Autodesk Inventor part; units mm, degrees
ref_plane "YZ Plane" through (0, 0, 0) normal (1, 0, 0) x (0, 1, 0)
ref_plane "XZ Plane" through (0, 0, 0) normal (0, 1, 0) x (-1, 0, 0)
ref_plane "XY Plane" through (0, 0, 0) normal (0, 0, 1) x (1, 0, 0)
sketch "Sketch1" plane through (0, 0, 0) normal (0, 1, 0) x (-1, 0, 0)
  line L0 (-11, 8) -> (11, 8)
  line L1 (11, 8) -> (11, -8)
  line L2 (11, -8) -> (-11, -8)
  line L3 (-11, -8) -> (-11, 8)
  line L4 (-11, 8) -> (11, -8) construction
  line L5 (11, 8) -> (-11, -8) construction
  point P0 (0, 0)
  dimension "d0" = 22
  dimension "d1" = 16
extrude "Extrusion1" add sketch "Sketch1" along normal blind 13
sketch "Sketch2" plane through (11, 0, 8) normal (1, 0, 0) x (0, 0, -1)
  line L0 (1.5, 11.7761) -> (14.5, 11.7761)
  line L1 (14.5, 11.7761) -> (14.5, 3.7761)
  line L2 (14.5, 3.7761) -> (1.5, 3.7761)
  line L3 (1.5, 3.7761) -> (1.5, 11.7761)
  line L4 (0, 0) -> (0, 13)
  line L5 (6.3059, 3.7761) -> (10.1899, 3.7761)
  line L6 (10.1899, 3.7761) -> (10.1899, 0.7851)
  line L7 (10.1899, 0.7851) -> (6.3059, 0.7851)
  line L8 (6.3059, 0.7851) -> (6.3059, 3.7761)
  point P0 (8, 0)
  dimension "d4" = 13
  dimension "d5" = 8
  dimension "d6" = 1.5
extrude "Extrusion2" cut sketch "Sketch2" against normal blind 16
properties part number "netwerk"
Design review of the part built by this model. Coordinates are the model's own, in mm. A direction names the side the tool comes from. Coordinates: 2 decimals unless noted, no trailing zeros. Loops run counter-clockwise (first coordinate to the right, second up) from the corner with the lowest first, then second, coordinate; pieces in that order, holes last. Notation, with made-up numbers: M -17,82 L 8,82 A20 ccw 8,86 Z; hole C 65.25,64 d6. An arc over 180 degrees is marked long. Answer as CSV lines item,"result".
Item 1: Add section A-A on x = 9.5. State the section outline as (y, z) points, plus the area to 3 significant figures.
Answer list:
outline,"M 0,-8 L 13,-8 L 13,8 L 0,8 Z; hole M 0.79,-2.19 L 3.78,-2.19 L 3.78,-6.5 L 11.78,-6.5 L 11.78,6.5 L 3.78,6.5 L 3.78,1.69 L 0.79,1.69 Z"
area,"92.4 mm²"
Item 2: For P1, Ø3.5, axis at y = 5.5, z = 0, coming from the +X side, flat-tipped, find the tip position at first contact; note if it passes through.
Answer list:
P1,"x = -5"
Item 3: Machinability: for faces 4 (the face through (3, 8, 6.5)), 5 (the face through (-11, 6, 0)), which of the approach directions +Z, -Z, +X, -X, +Y, -Y give a long, thin tool a straight path to every point of the face, cutting with its end or side? Answer none if there is none.
Answer list:
face 4,"+X"
face 5,"+Z, -Z, -X, +Y, -Y"
Item 4: For probe 1 along Y at (x, z) = (2.25, -1); probe 2 along Z at (x, y) = (-2.5, 1.5); probe 3 along Y at (x, z) = (-2.75, 3.75), list the stretches that pass through material, from the lowest coordinate up.
Answer list:
probe 1,"0 to 0.79, 11.78 to 13"
probe 2,"-8 to -2.19, 1.69 to 8"
probe 3,"0 to 3.78, 11.78 to 13"
Item 5: Add section C-C on y = 2. State the section outline as (x, z) points.
Answer list:
outline,"M -11,-8 L 11,-8 L 11,-2.19 L -5,-2.19 L -5,1.69 L 11,1.69 L 11,8 L -11,8 Z"
Item 6: Add section B-B on z = 1. State the section outline as (x, y) points.
Answer list:
outline,"M -11,0 L 11,0 L 11,0.79 L -5,0.79 L -5,11.78 L 11,11.78 L 11,13 L -11,13 Z"
Item 7: The part is to be moulded in two halves that separate along Y. For faces 1 (the face through (0, 0, 0)), 2 (the face through (3, 3.776, -4)), 3 (the face through (0, 13, 0)), say which applies: pulls with the +Y half, pulls with the -Y half, needs draft (parallel to the pull), parting line crosses it, or undercut.
Answer list:
face 1,"pulls with the -Y half"
face 2,"undercut"
face 3,"pulls with the +Y half"
